Can you work these out from the drawing? Everything is in mm from the part's minimum corner. A direction names the side the tool comes from. Coordinates: 2 decimals unless noted, no trailing zeros. Loops run counter-clockwise (first coordinate to the right, second up) from the corner with the lowest first, then second, coordinate; pieces in that order, holes last.
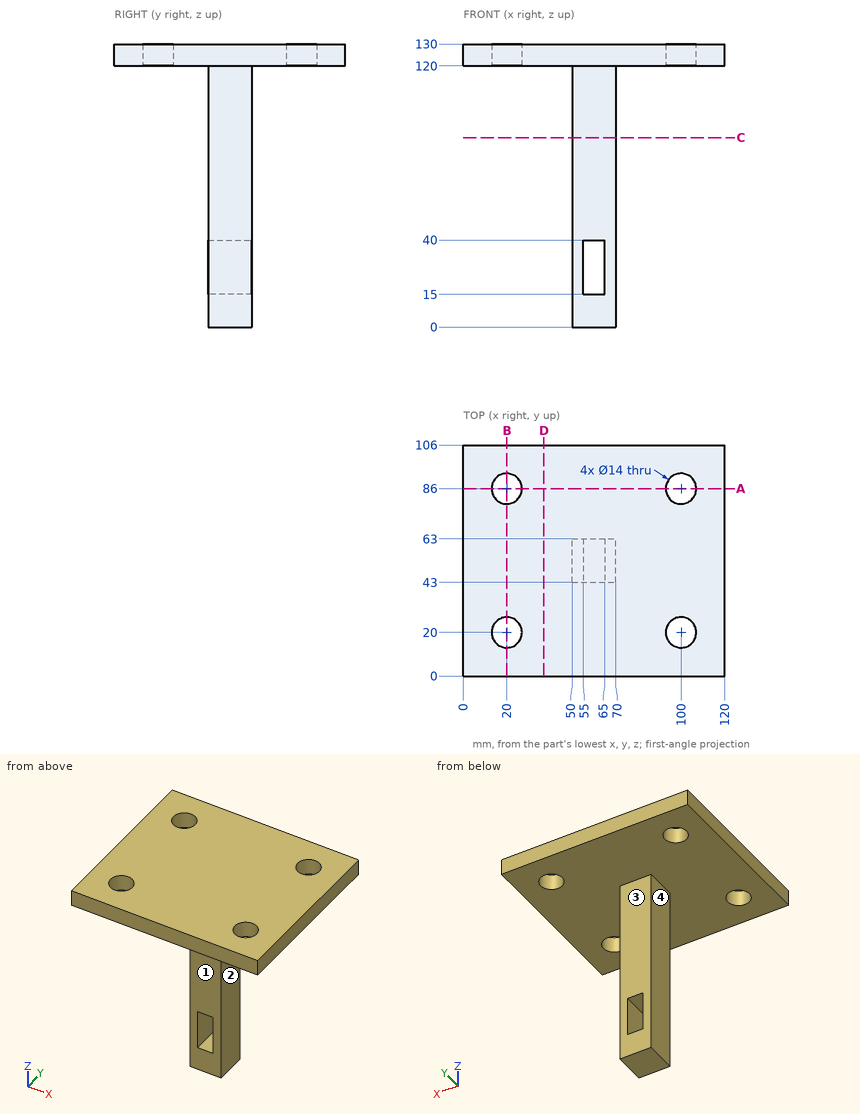
(1) Imagine slicing it at B-B, the plane x = 20. Write out the boundary of the cut face in (y, z).
Answers:
outline: (0, 120) - (13, 120) - (13, 130) - (0, 130) - close; (27, 120) - (79, 120) - (79, 130) - (27, 130) - close; (93, 120) - (106, 120) - (106, 130) - (93, 130) - close
(2) For pin 1 (16 mm diameter, centred on x = 59.5, z = 74.5, fed in from +Y); pin 2 (12 mm diameter, centred on y = 50, z = 95.5, fed in from -X); pin 3 (16 mm diameter, centred on y = 49, z = 27.5, fed in from +X), each with a flat end and sliding along its axis, tell me the tip position at first contact or that it passes through.
Answers:
pin 1: stops at y = 63
pin 2: stops at x = 50
pin 3: stops at x = 70
(3) Imagine slicing it at A-A, the plane y = 86. Write out the boundary of the cut face in (x, z), and give its area (3 significant figures).
Answers:
outline: (0, 120) - (13, 120) - (13, 130) - (0, 130) - close; (27, 120) - (93, 120) - (93, 130) - (27, 130) - close; (107, 120) - (120, 120) - (120, 130) - (107, 130) - close
area: 920 mm2
(4) Imagine slicing it at D-D, the plane x = 37. Write out the boundary of the cut face in (y, z).
Answers:
outline: (0, 120) - (106, 120) - (106, 130) - (0, 130) - close
(5) Which directions (+Z, -Z, +X, -X, +Y, -Y) give clear straight access to the entire face, cutting with the end or side of a thin tool? Please do the marked faces 1, 2, 3 and 4.
Answers:
face 1: -Z, +X, -X, -Y
face 2: -Z, +X, +Y, -Y
face 3: -Z, +X, -X, +Y
face 4: -Z, -X, +Y, -Y
(6) Imagine slicing it at C-C, the plane z = 87. Write out the boundary of the cut face in (x, y), and give its area (3 significant figures).
Answers:
outline: (50, 43) - (70, 43) - (70, 63) - (50, 63) - close
area: 400 mm2
(7) I need wall thicknesses on probe 1 along Y at (x, z) = (20, 122.5); probe 2 along Z at (x, y) = (56, 92); probe 3 along Y at (x, z) = (53, 62). Which ranges of each line are inside material? Lowest first, please.
Answers:
probe 1: y = 0 to 13, 27 to 79, 93 to 106
probe 2: z = 120 to 130
probe 3: y = 43 to 63
